Verification items for the finished model (mm, model axes). A direction names the side the tool comes from. Coordinates: 2 decimals unless noted, no trailing zeros. Order: outer loops, then holes, each group sorted by start corner. A loop starts at its lowest first (then second) coordinate and runs counter-clockwise, first axis right, second up. Notation, with made-up numbers: (-12, -40) -> (47, -40) arc R31 ccw to (47, -13) -> close; hole circle Ø9 at (53.5, -8). An arc over 180 degrees is marked (long way). Answer as CSV lines item,"result".
```python
from build123d import *

# Parameters (mm, degrees)
BOSS_EXTRUDE1_DEPTH = 40
SKETCH3_R           = 7.5
SKETCH3_R_2         = 2.25
CUT_EXTRUDE1_DEPTH  = 3
SKETCH4_R           = 7.5
SKETCH4_R_2         = 2.25
CUT_EXTRUDE2_DEPTH  = 3
SKETCH5_R           = 7.5
SKETCH5_R_2         = 2.25
CUT_EXTRUDE3_DEPTH  = 3
SKETCH6_R           = 7.5
SKETCH6_R_2         = 2.25
CUT_EXTRUDE4_DEPTH  = 3
SKETCH7_R           = 7.5
SKETCH7_R_2         = 2.25
CUT_EXTRUDE5_DEPTH  = 3
BOSS_EXTRUDE2_DEPTH = 3


with BuildPart() as part:
    # Sketch2 → Boss-Extrude1 (new body)
    with BuildSketch(Plane(origin=(0, 0, 0), x_dir=(1, 0, 0), z_dir=(0, 1, 0))):
        Polygon((18.889370654, -26.231276984), (30.784563452, 9.858948677), (0.136535888, 32.32444236), (-30.700179633, 10.118655369), (-19.110290361, -26.070769422), align=None)
    extrude(amount=BOSS_EXTRUDE1_DEPTH)

    # Sketch3 → Cut-Extrude1 (cut)
    with BuildSketch(Plane(origin=(-0.110459853, 0, 26.151023203), x_dir=(0.999991079365483, 0, 0.004223883220016987), z_dir=(-0.004223883220016987, 0, 0.9999910793654831))):
        with Locations((0, 20)):
            Circle(SKETCH3_R)
        with Locations((-16, 20)):
            Circle(SKETCH3_R_2)
    extrude(amount=-CUT_EXTRUDE1_DEPTH, mode=Mode.SUBTRACT)

    # Sketch4 → Cut-Extrude2 (cut)
    with BuildSketch(Plane(origin=(24.836967053, 0, 8.186164153), x_dir=(0.3130313894077477, 0, -0.9497427805703264), z_dir=(0.9497427805703265, 0, 0.3130313894077478))):
        with Locations((0, 20)):
            Circle(SKETCH4_R)
        with Locations((-16, 20)):
            Circle(SKETCH4_R_2)
    extrude(amount=-CUT_EXTRUDE2_DEPTH, mode=Mode.SUBTRACT)

    # Sketch5 → Cut-Extrude3 (cut)
    with BuildSketch(Plane(origin=(15.46054967, 0, -21.091695519), x_dir=(-0.8065270411658909, 0, -0.591197202182312), z_dir=(0.5911972021823119, 0, -0.8065270411658908))):
        with Locations((0, 20)):
            Circle(SKETCH5_R)
        with Locations((-16, 20)):
            Circle(SKETCH5_R_2)
    extrude(amount=-CUT_EXTRUDE3_DEPTH, mode=Mode.SUBTRACT)

    # Sketch6 → Cut-Extrude4 (cut)
    with BuildSketch(Plane(origin=(-15.281821873, 0, -21.221548864), x_dir=(-0.8114925136941543, 0, 0.584362815567814), z_dir=(-0.5843628155678139, 0, -0.8114925136941542))):
        with Locations((0, 20)):
            Circle(SKETCH6_R)
        with Locations((-16, 20)):
            Circle(SKETCH6_R_2)
    extrude(amount=-CUT_EXTRUDE4_DEPTH, mode=Mode.SUBTRACT)

    # Sketch7 → Cut-Extrude5 (cut)
    with BuildSketch(Plane(origin=(-24.905234997, 0, 7.976057027), x_dir=(0.304997086086814, 0, 0.9523532839648071), z_dir=(-0.9523532839648071, 0, 0.304997086086814))):
        with Locations((0, 20)):
            Circle(SKETCH7_R)
        with Locations((-16, 20)):
            Circle(SKETCH7_R_2)
    extrude(amount=-CUT_EXTRUDE5_DEPTH, mode=Mode.SUBTRACT)

    # Sketch8 → Boss-Extrude2 (add)
    with BuildSketch(Plane.XZ):
        Polygon((30.784563452, -9.858948677), (18.889370654, 26.231276984), (-19.110290361, 26.070769422), (-30.700179633, -10.118655369), (0.136535888, -32.32444236), align=None)
    extrude(amount=BOSS_EXTRUDE2_DEPTH)


solid = part.part
```
Item 1: Release check for a two-part mould opening along Y. For faces 3 (the flat face through (-22.25, 18.8, 16.27)), 4 (the flat face through (26.62, 20.03, -9.19)) record: +Y half, -Y half, draft (parallel to the pull), parting line (faces both ways), or undercut.
Answer list:
face 3,"draft"
face 4,"undercut"
Item 2: Section check B-B, the plane y = 9.5. Record the boundary of the cut face in (x, z), plus the area to 3 significant figures.
Answer list:
outline,"(-30.7, -10.12) -> (0.14, -32.32) -> (30.78, -9.86) -> (18.89, 26.23) -> (-19.11, 26.07) -> close"
area,"2,480 mm2"
Item 3: Section check C-C, the plane z = -4. Record the boundary of the cut face in (x, y).
Answer list:
outline,"(-28.74, -3) -> (28.85, -3) -> (28.85, 40) -> (-28.74, 40) -> close"
Item 4: Section check A-A, the plane y = 24.5. Record the boundary of the cut face in (x, z), plus the area to 3 significant figures.
Answer list:
outline,"(-30.7, -10.12) -> (-20.15, -17.72) -> (-18.4, -15.28) -> (-8.66, -22.29) -> (-10.41, -24.73) -> (0.14, -32.32) -> (10.62, -24.64) -> (8.85, -22.22) -> (18.53, -15.12) -> (20.3, -17.54) -> (30.78, -9.86) -> (26.72, 2.49) -> (23.87, 1.55) -> (20.11, 12.95) -> (22.96, 13.88) -> (18.89, 26.23) -> (5.89, 26.18) -> (5.9, 23.18) -> (-6.1, 23.13) -> (-6.11, 26.13) -> (-19.11, 26.07) -> (-23.08, 13.69) -> (-20.22, 12.78) -> (-23.88, 1.35) -> (-26.74, 2.26) -> close"
area,"2,300 mm2"
Item 5: Tool access check on faces 1 (the flat face through (16.97, 20.03, 22.47)), 2 (the flat face through (-22.35, 18.8, -16.13)). Record the directions out of +Z, -Z, +X, -X, +Y, -Y that give a thin tool (end or side, any length) a straight path to the whole face; none if there is none.
Answer list:
face 1,"none"
face 2,"-Z, -X, +Y, -Y"
Item 6: Depth check by flat-ended pin: pin 1 Ø12 at (y, z) = (18, 15.5) entering from -X; pin 2 Ø6 at (y, z) = (32.5, -5.5) entering from +X; pin 3 Ø2 at (x, y) = (-5, 12) entering from -Z. Enter the tip coordinate at first touch or a pass-through.
Answer list:
pin 1,"x = -23.77"
pin 2,"x = 30.34"
pin 3,"z = -29.35"
Item 7: Thickness scan on line 1 (X direction, y = 37.5, z = 5); line 2 (X direction, y = 10, z = -12); line 3 (Y direction, x = 19, z = 22). Record the ranges inside material, lowest first.
Answer list:
line 1,"-25.86 to 25.89"
line 2,"-28.09 to 27.86"
line 3,"-3 to 18.01, 21.99 to 40"
